from build123d import *

# Parameters (mm, degrees)
F0_R     = 15.5
F1_DEPTH = 14
F2_W     = 36
F2_H     = 1.65
F3_DEPTH = 8.6
F4_W     = 1.6
F4_H     = 40
F5_DEPTH = 8.6
F6_R     = 5.6
F7_DEPTH = 9
F8_SIZE  = 0.8
F9_SIZE  = 0.5


with BuildPart() as f1:
    # F0 (on Front) → F1 (new body)
    with BuildSketch(Plane.XZ):
        Circle(F0_R)
        with BuildLine():
            ThreePointArc((3.011229, 1.35), (0, -3.3), (-3.011229, 1.35))
            Line((-3.011229, 1.35), (3.011229, 1.35))
        make_face(mode=Mode.SUBTRACT)
    extrude(amount=F1_DEPTH)

    # F2 (on Front) → F3 (cut)
    with BuildSketch(Plane.XZ):
        Rectangle(F2_W, F2_H)
    extrude(amount=F3_DEPTH, mode=Mode.SUBTRACT)

    # F4 (on Front) → F5 (cut)
    with BuildSketch(Plane.XZ):
        Rectangle(F4_W, F4_H)
    extrude(amount=F5_DEPTH, mode=Mode.SUBTRACT)

    # F6 (on Front) → F7 (cut)
    with BuildSketch(Plane.XZ):
        Circle(F6_R)
    extrude(amount=F7_DEPTH, mode=Mode.SUBTRACT)

    # F8
    f8_edges = [f1.edges().sort_by_distance(p)[0] for p in [
        (0, -14, 1.35),
        (0, -14, -3.3),
    ]]
    chamfer(f8_edges, length=F8_SIZE)

    # F9
    f9_edges = [f1.edges().sort_by_distance(p)[0] for p in [
        (10.508463, 0, 0.825),
        (-10.508463, 0, 0.825),
        (-10.508463, 0, -0.825),
        (10.508463, 0, -0.825),
        (-0.8, 0, 10.510952),
        (-0.8, 0, -10.510952),
        (0.8, 0, 10.510952),
        (0.8, 0, -10.510952),
        (3.950855, 0, 3.968721),
        (-3.950855, 0, 3.968721),
        (-3.950855, 0, -3.968721),
        (3.950855, 0, -3.968721),
        (10.951301, 0, 10.969003),
        (-10.951301, 0, 10.969003),
        (-10.951301, 0, -10.969003),
        (10.951301, 0, -10.969003),
    ]]
    chamfer(f9_edges, length=F9_SIZE)


solid = f1.part
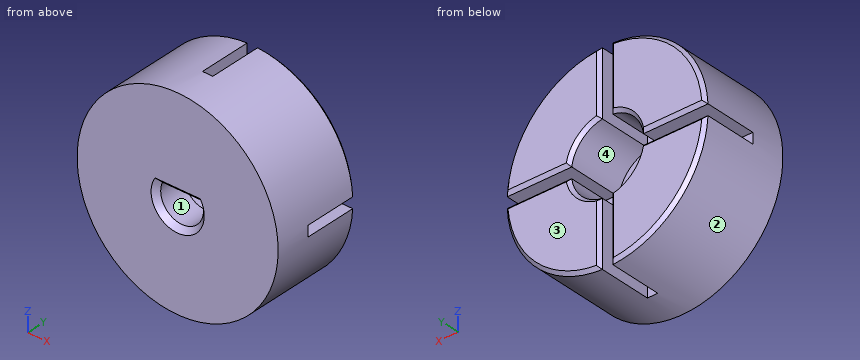
Input: part model. Units: mm. Frame: model coordinates. Face numbers are marked on the shaded views. Round coordinates to 2 decimals unless told otherwise and drop trailing zeros. Loops run counter-clockwise (first coordinate to the right, second up) from the corner with the lowest first, then second, coordinate; pieces in that order, holes last. Notation, with made-up numbers: (67.5, 75) -> (89.5, 75) arc R32 cw to (89.5, 105) -> close; hole circle Ø10 at (33, 81.5). An arc over 180 degrees is marked (long way). Answer as a JSON object with one key per item and string values. Group by question number.
1) Ray query, L1, parallel to Z at x = 0, y = -12.2; L2, parallel to X at y = -10.4, z = 0. Return the intervals inside material, ascending.
2) Section query A-A on y = -5.25. Output: boundary loops of the cut face in (x, z) (3 decimals), plus the area to 3 significant figures.
3) Section query C-C on y = -9.5. Output: boundary loops of the cut face in (x, z), plus the area to 3 significant figures.
4) Pin query (flat end, axial travel): pin 1 (3 mm diameter, centred on x = 4, y = -1.5, fed in from +Z); pin 2 (3 mm diameter, centred on y = -5, z = 2, fed in from +X); pin 3 (2 mm diameter, centred on y = -6, z = -12, fed in from +X). Return the tip coordinate at first contact, or that it passes through.
5) Section query B-B on x = 0. Output: boundary loops of the cut face in (y, z).
6) Draft query along X for the marked faces 1, 2, 3 and 4. Return one class per face: +X half, -X half, draft (parallel to the pull), parting line (faces both ways), or undercut.
Reply:
{
 "1": {"L1": "z = -15.5 to -3.3, 1.35 to 15.5", "L2": "x = -15.5 to -3.3, 3.3 to 15.5"},
 "2": {"outline": "(-15.478, -0.825) arc R15.5 ccw to (-0.8, -15.479) -> (-0.8, -5.543) arc R5.6 cw to (-5.539, -0.825) -> close; (-15.478, 0.825) -> (-5.539, 0.825) arc R5.6 cw to (-0.8, 5.543) -> (-0.8, 15.479) arc R15.5 ccw to start; (0.8, -15.479) arc R15.5 ccw to (15.478, -0.825) -> (5.539, -0.825) arc R5.6 cw to (0.8, -5.543) -> close; (0.8, 5.543) arc R5.6 cw to (5.539, 0.825) -> (15.478, 0.825) arc R15.5 ccw to (0.8, 15.479) -> close", "area": "592 mm2"},
 "3": {"outline": "circle Ø31 at (0, 0); hole (-3.01, 1.35) arc R3.3 ccw (long way) to (3.01, 1.35) -> close", "area": "729 mm2"},
 "4": {"pin 1": "stops at z = 15.3", "pin 2": "stops at x = 15.48", "pin 3": "stops at x = 10.92"},
 "5": {"outline": "(-14, -15.5) -> (-8.6, -15.5) -> (-8.6, -5.6) -> (-9, -5.6) -> (-9, -3.3) -> (-13.2, -3.3) -> (-14, -4.1) -> close; (-14, 2.15) -> (-13.2, 1.35) -> (-9, 1.35) -> (-9, 5.6) -> (-8.6, 5.6) -> (-8.6, 15.5) -> (-14, 15.5) -> close"},
 "6": {"face 1": "undercut", "face 2": "parting line", "face 3": "draft", "face 4": "undercut"}
}
